Geometry check sheet. Reference: drawing and pictorial views, mm from the part's lowest x, y, z. A direction names the side the tool comes from. Give positions to 0.01 mm unless a question says otherwise; leave off trailing zeros. Order: outer loops, then holes, each group sorted by start corner. A loop starts at its lowest first (then second) coordinate and runs counter-clockwise, first axis right, second up.
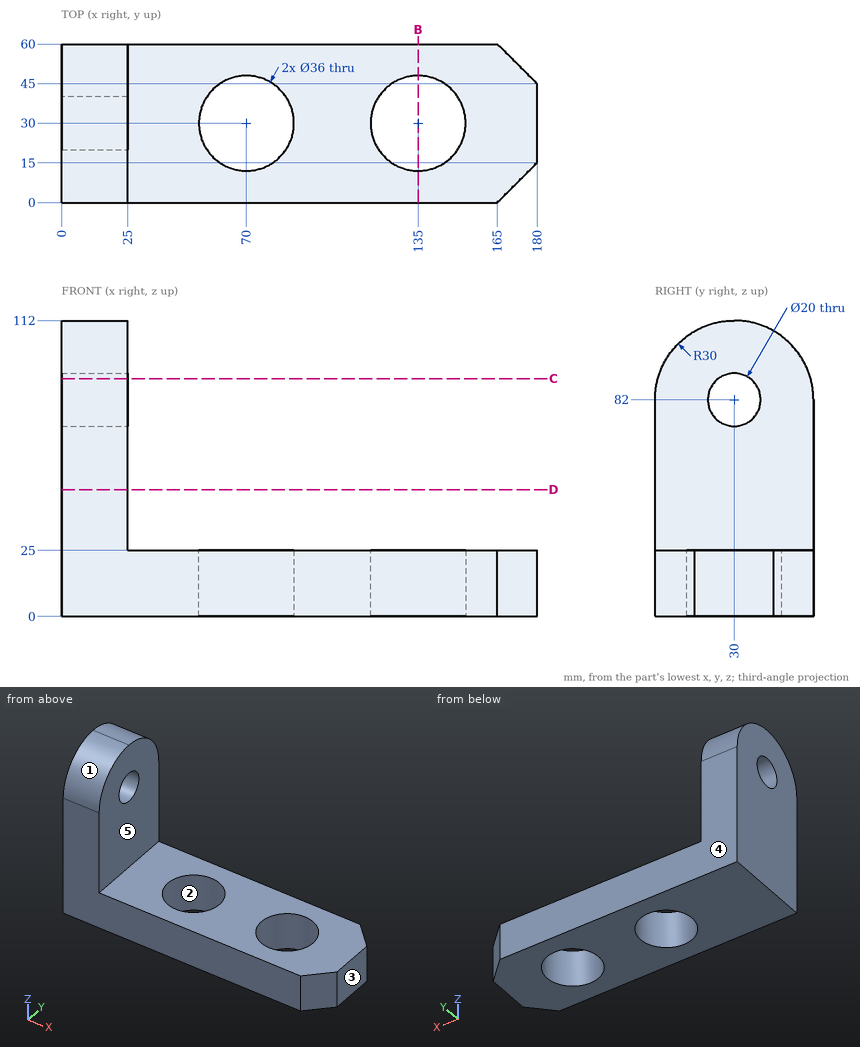
1) Set-up check for the marked faces 4 and 5: record each of +Z, -Z, +X, -X, +Y, -Y from which the full face is reachable in a straight line by a thin tool's end or side.
Recorded:
face 4: +Z, -Z, +X, -X, +Y
face 5: +Z, +X, +Y, -Y
2) Draft check along X on the marked faces 1, 2 and 3. Enter one of: +X half, -X half, draft (parallel to the pull), parting line (faces both ways), or undercut.
Recorded:
face 1: draft
face 2: undercut
face 3: +X half
3) Depth check by flat-ended pin: pin 1 Ø10 at (y, z) = (6, 72) entering from +X; pin 2 Ø12 at (y, z) = (30, 82) entering from +X; pin 3 Ø1.5 at (y, z) = (24.5, 14.5) entering from -X. Enter the tip coordinate at first touch or a pass-through.
Recorded:
pin 1: stops at x = 25
pin 2: passes through
pin 3: stops at x = 0
4) Section check C-C, the plane z = 90. Record the cut outline in (x, y).
Recorded:
outline: (0, 1.09) - (25, 1.09) - (25, 24) - (0, 24) - close; (0, 36) - (25, 36) - (25, 58.91) - (0, 58.91) - close
5) Material ranges on L1, parallel to Z at x = 18, y = 30; L2, parallel to Y at x = 135, z = 8.5; L3, parallel to X at y = 43, z = 15.5, recorded low to high.
Recorded:
L1: z = 0 to 72, 92 to 112
L2: y = 0 to 12, 48 to 60
L3: x = 0 to 57.55, 82.45 to 122.55, 147.45 to 180
6) Section check B-B, the plane x = 135. Record the cut outline in (y, z).
Recorded:
outline: (0, 0) - (12, 0) - (12, 25) - (0, 25) - close; (48, 0) - (60, 0) - (60, 25) - (48, 25) - close
7) Section check D-D, the plane z = 48. Record the cut outline in (x, y).
Recorded:
outline: (0, 0) - (25, 0) - (25, 60) - (0, 60) - close
